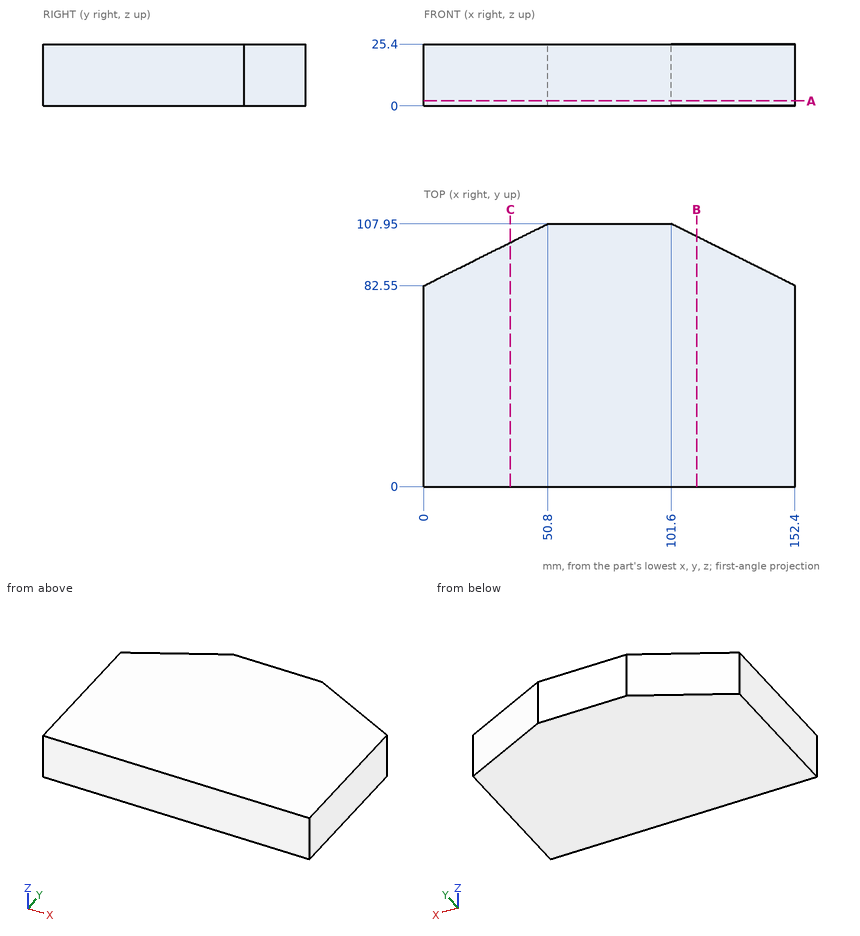
Could you check a few things on this drawing? It's one solid part, dimensions in mm from its lowest x, y, z. Coordinates: 2 decimals unless noted, no trailing zeros. Order: outer loops, then holes, each group sorted by start corner. A loop starts at its lowest first (then second) coordinate and runs counter-clockwise, first axis right, second up. Notation, with made-up numbers: (-14.5, 42.5) - (18.5, 42.5) arc R27 ccw to (18.5, 71.5) - close; hole circle Ø8 at (24.25, -40). An arc over 180 degrees is marked (long way). One line per question, with ' | ' between items. Start each with the question number.
1. If we section it at C-C (x = 35.5): Write out the boundary of the cut face in (y, z), and give its area (3 significant figures).
2. If we section it at A-A (z = 2): Write out the boundary of the cut face in (x, y), and give its area (3 significant figures).
3. Please list where these lines run through material, in increasing order: line 1 along Y through (x, z) = (138, 1); line 2 along Y through (x, z) = (105, 8.25); line 3 along X through (y, z) = (103.5, 3). Write a range as [from, to].
4. I'm going to push flat-ended pins straight in: pin 1 Ø1.5 at (x, z) = (45, 12) entering from -Y; pin 2 Ø5 at (y, z) = (87, 22.5) entering from -X. Where does each tip first touch, or does it pass through?
5. If we section it at B-B (x = 112): Write out the boundary of the cut face in (y, z), and give its area (3 significant figures).
Model answer:
1) outline: (0, 0) - (100.3, 0) - (100.3, 25.4) - (0, 25.4) - close | area: 2,550 mm²
2) outline: (0, 0) - (152.4, 0) - (152.4, 82.55) - (101.6, 107.95) - (50.8, 107.95) - (0, 82.55) - close | area: 15,200 mm²
3) line 1: y = [0, 89.75] | line 2: y = [0, 106.25] | line 3: x = [41.9, 110.5]
4) pin 1: stops at y = 0 | pin 2: stops at x = 3.9
5) outline: (0, 0) - (102.75, 0) - (102.75, 25.4) - (0, 25.4) - close | area: 2,610 mm²
